Can you work these out from the model? Positions are in its coordinate system, mm. A direction names the side the tool comes from. Give positions to 0.01 mm unless a question says otherwise; leave off trailing zeros. Order: outer loops, then holes, each group sorted by start corner. A loop starts at its lowest first (then second) coordinate and runs counter-clockwise, first axis right, second up. Notation, with made-up numbers: (58.25, -17.75) - (97.25, -17.75) arc R18 ccw to (97.25, 6.25) - close; hole circle Ø5 at (-25.5, 8.25). An arc over 180 degrees is marked (long way). Use one line per item in the form item = value. Start each with the question number.
1) Please list where these lines run through material, in increasing order: probe 1 along Z at (x, y) = (0, 2.1) (3 decimals); probe 2 along Z at (x, y) = (-1.25, 5); probe 3 along Y at (x, z) = (-2.5, -1.5).
2) Which directions (+Z, -Z, +X, -X, +Y, -Y) give clear straight access to the entire face, cutting with the end or side of a thin tool? Please do faces 3 (the cylindrical face through (-0.28, 20.22, 2.14)), 4 (the cylindrical face through (-2.217, 10.966, -1.7)), 5 (the cylindrical face through (-0.385, 11.132, -1.736)).
3) Suppose I cut it at C-C, the plane y = 2.5. Write out the boundary of the cut face in (x, z) (3 decimals), and give its area (3 significant figures).
4) For pin 1 (3 mm diameter, centred on x = 0, z = 0, fed in from +Y); pin 2 (3 mm diameter, centred on y = 6.5, z = -2, fed in from -X); pin 3 (3 mm diameter, centred on x = -1.5, z = 2, fed in from -Y), each with a flat end and sliding along its axis, tell me the tip position at first contact or that it passes through.
5) We'd pull the mould along X, two halves only. Please class faces 1 (the cylindrical face through (-0.28, 1.93, 2.14)), 2 (the cylindrical face through (-0.69, 1.88, -3.1)): released by +X, released by -X, zero draft, split by the parting line, or undercut.
6) Suppose I cut it at D-D, the plane y = 17.25. Write out the boundary of the cut face in (x, z).
```python
from build123d import *


with BuildPart() as part:
    # Sketch1 → Revolve-Thin1 (revolve)
    with BuildSketch(Plane.XY):
        with BuildLine():
            Line((3.175, 22.098), (3.175, 18.288))
            ThreePointArc((3.175, 18.288), (3.126446888, 17.940196176), (2.9845, 17.618985987))
            ThreePointArc((2.9845, 17.618985987), (2.842553112, 17.297775797), (2.794, 16.949971973))
            Line((2.794, 16.949971973), (2.794, 5.148028027))
            ThreePointArc((2.794, 5.148028027), (2.842553112, 4.800224203), (2.9845, 4.479014013))
            ThreePointArc((2.9845, 4.479014013), (3.126446888, 4.157803824), (3.175, 3.81))
            Line((3.175, 3.81), (3.175, 0))
            Line((3.175, 0), (2.159, 0))
            Line((2.159, 0), (2.159, 3.81))
            ThreePointArc((2.159, 3.81), (2.149289378, 3.879560765), (2.1209, 3.943802803))
            ThreePointArc((2.1209, 3.943802803), (1.865395602, 4.521981143), (1.778, 5.148028027))
            Line((1.778, 5.148028027), (1.778, 16.949971973))
            ThreePointArc((1.778, 16.949971973), (1.865395602, 17.576018857), (2.1209, 18.154197197))
            ThreePointArc((2.1209, 18.154197197), (2.149289378, 18.218439235), (2.159, 18.288))
            Line((2.159, 18.288), (2.159, 22.098))
            Line((2.159, 22.098), (3.175, 22.098))
        make_face()
    revolve(axis=Axis((0, 22.098, 0), (0, -1, 0)))


solid = part.part
```
Result sheet:
q1.probe_1 = -3.175 to -2.159, 2.159 to 3.175
q1.probe_2 = -2.51 to -1.27, 1.27 to 2.51
q1.probe_3 = 0 to 4.61, 17.49 to 22.1
q2.face_3 = +Y
q2.face_4 = none
q2.face_5 = +Y, -Y
q3.outline = circle Ø6.35 at (0, 0); hole circle Ø4.318 at (0, 0)
q3.area = 17.0 mm²
q4.pin_1 = through
q4.pin_2 = -2.75
q4.pin_3 = 0
q5.face_1 = undercut
q5.face_2 = split by the parting line
q6.outline = circle Ø5.66 at (0, 0); hole circle Ø3.6 at (0, 0)
